from build123d import *

# Parameters (mm, degrees)
SKETCH1_R            = 1.5
BOSS_EXTRUDE1_DEPTH  = 2
SKETCH2_R            = 2
BOSS_EXTRUDE2_DEPTH  = 0.5
SKETCH3_W            = 5
SKETCH3_H            = 5
BOSS_EXTRUDE3_DEPTH  = 10.5
SKETCH4_R            = 1.9
BOSS_EXTRUDE4_DEPTH  = 3.5
BOSS_EXTRUDE5_DEPTH  = 2.5
BOSS_EXTRUDE9_DEPTH  = 2
SKETCH8_R            = 2
BOSS_EXTRUDE10_DEPTH = 5
BOSS_EXTRUDE12_START = -3.5
BOSS_EXTRUDE12_DEPTH = 3.5
CUT_EXTRUDE1_START   = -3.5
CUT_EXTRUDE1_DEPTH   = 3.5
CUT_EXTRUDE4_START   = -2.25
CUT_EXTRUDE4_DEPTH   = 2.25
SKETCH14_R           = 2
SKETCH14_R_2         = 1.5
CUT_EXTRUDE5_DEPTH   = 3.25
BOSS_EXTRUDE13_START = 0.5
SKETCH15_R           = 2
SKETCH15_R_2         = 1.5
BOSS_EXTRUDE13_DEPTH = 0.5
BOSS_EXTRUDE14_START = 0.5
SKETCH17_R           = 1.5
BOSS_EXTRUDE14_DEPTH = 0.5


# Read off the part's stored shape, not the designer's step: Cut-Extrude4
with BuildPart() as part:
    # Sketch1 → Boss-Extrude1 (new body)
    with BuildSketch(Plane(origin=(0, 0, 0), x_dir=(1, 0, 0), z_dir=(0, 1, 0))):
        with Locations(Location((0, 0, 0), (0, 0, 270))):
            Circle(SKETCH1_R)
    extrude(amount=BOSS_EXTRUDE1_DEPTH)

    # Sketch2 → Boss-Extrude2 (add)
    with BuildSketch(Plane(origin=(0, 2, 0), x_dir=(1, 0, 0), z_dir=(0, 1, 0))):
        with Locations(Location((0, 0, 0), (0, 0, 270))):
            Circle(SKETCH2_R)
    extrude(amount=BOSS_EXTRUDE2_DEPTH)

    # Sketch3 → Boss-Extrude3 (add)
    with BuildSketch(Plane(origin=(0, 2.5, 0), x_dir=(1, 0, 0), z_dir=(0, 1, 0))):
        Rectangle(SKETCH3_W, SKETCH3_H)
    extrude(amount=BOSS_EXTRUDE3_DEPTH)

    # Sketch4 → Boss-Extrude4 (add)
    with BuildSketch(Plane(origin=(0, 13, 0), x_dir=(1, 0, 0), z_dir=(0, 1, 0))):
        with Locations(Location((0, 0, 0), (0, 0, 270))):
            Circle(SKETCH4_R)
    extrude(amount=BOSS_EXTRUDE4_DEPTH)

    # Sketch5 → Boss-Extrude5 (add)
    with BuildSketch(Plane(origin=(0, 16.5, 0), x_dir=(1, 0, 0), z_dir=(0, 1, 0))):
        with BuildLine():
            Line((1.549193338, -1.1), (-1.549193338, -1.1))
            ThreePointArc((-1.549193338, -1.1), (0, 1.9), (1.549193338, -1.1))
        make_face()
    extrude(amount=BOSS_EXTRUDE5_DEPTH)

    # Sketch7 → Boss-Extrude9 (add)
    with BuildSketch(Plane(origin=(2.5, 0, 0), x_dir=(0, 0, -1), z_dir=(1, 0, 0))):
        with BuildLine():
            ThreePointArc((-2.5, 3.469223594), (-2.090990258, 2.909009742), (-1.530776406, 2.5))
            Line((-1.530776406, 2.5), (0.530776406, 2.5))
            ThreePointArc((0.530776406, 2.5), (1.090990258, 6.090990258), (-2.5, 5.530776406))
            Line((-2.5, 5.530776406), (-2.5, 3.469223594))
        make_face()
    boss_extrude9 = extrude(amount=BOSS_EXTRUDE9_DEPTH)

    # Sketch8 → Boss-Extrude10 (add)
    with BuildSketch(Plane(origin=(4.5, 0, 0), x_dir=(0, 0, -1), z_dir=(1, 0, 0))):
        with Locations(Location((-0.5, 4.5, 0), (0, 0, 180))):
            Circle(SKETCH8_R)
    boss_extrude10 = extrude(amount=BOSS_EXTRUDE10_DEPTH)

    # Mirror1: Boss-Extrude9, Boss-Extrude10 across plane
    add(boss_extrude9.mirror(Plane(origin=(0, 0, 0), x_dir=(0, 0, 1), z_dir=(1, 0, 0))))
    add(boss_extrude10.mirror(Plane(origin=(0, 0, 0), x_dir=(0, 0, 1), z_dir=(1, 0, 0))))

    # Sketch10 → Boss-Extrude12 (add)
    with BuildSketch(Plane(origin=(0, 16.5, 0), x_dir=(1, 0, 0), z_dir=(0, 1, 0)).offset(BOSS_EXTRUDE12_START)):
        with BuildLine():
            ThreePointArc((-1.549193338, -1.1), (0, -1.9), (1.549193338, -1.1))
            Line((1.549193338, -1.1), (-1.549193338, -1.1))
        make_face()
    extrude(amount=BOSS_EXTRUDE12_DEPTH)

    # Sketch11 → Cut-Extrude1 (cut)
    with BuildSketch(Plane(origin=(0, 16.5, 0), x_dir=(1, 0, 0), z_dir=(0, 1, 0)).offset(CUT_EXTRUDE1_START)):
        with BuildLine():
            Line((-1.549193338, -1.1), (1.549193338, -1.1))
            ThreePointArc((1.549193338, -1.1), (0, -1.9), (-1.549193338, -1.1))
        make_face()
    extrude(amount=CUT_EXTRUDE1_DEPTH, mode=Mode.SUBTRACT)

    # Cut-Extrude4 outline → Cut-Extrude4 (cut)
    with BuildSketch(Plane(origin=(9.5, 0, 0), x_dir=(0, 0, -1), z_dir=(1, 0, 0)).offset(CUT_EXTRUDE4_START)):
        with BuildLine():
            ThreePointArc((0.5, 2.767949192), (1.5, 4.5), (0.5, 6.232050808))
            Line((0.5, 6.232050808), (0.5, 2.767949192))
        make_face()
    extrude(amount=CUT_EXTRUDE4_DEPTH, mode=Mode.SUBTRACT)

    # Sketch14 → Cut-Extrude5 (cut)
    with BuildSketch(Plane.ZY.offset(9.5)):
        with Locations((0.5, 4.5)):
            Circle(SKETCH14_R)
        with Locations((0.5, 4.5)):
            Circle(SKETCH14_R_2, mode=Mode.SUBTRACT)
    extrude(amount=-CUT_EXTRUDE5_DEPTH, mode=Mode.SUBTRACT)

    # Sketch15 → Boss-Extrude13 (add)
    with BuildSketch(Plane.ZY.offset(6.25).offset(BOSS_EXTRUDE13_START)):
        with Locations((0.5, 4.5)):
            Circle(SKETCH15_R)
        with Locations((0.5, 4.5)):
            Circle(SKETCH15_R_2, mode=Mode.SUBTRACT)
    extrude(amount=-BOSS_EXTRUDE13_DEPTH)

    # Sketch17 → Boss-Extrude14 (add)
    with BuildSketch(Plane.ZY.offset(9.5).offset(BOSS_EXTRUDE14_START)):
        with Locations((0.5, 4.5)):
            Circle(SKETCH17_R)
    extrude(amount=-BOSS_EXTRUDE14_DEPTH)


solid = part.part
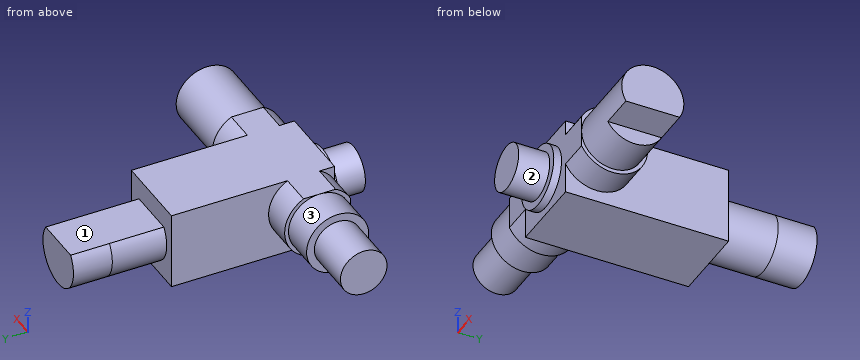
Read the model definition and answer for the solid it produces. Units are mm, in the model's axes. Face numbers are marked on the shaded views. A direction names the side the tool comes from. Round coordinates to 2 decimals unless told otherwise and drop trailing zeros. Order: outer loops, then holes, each group sorted by start corner. A loop starts at its lowest first (then second) coordinate and runs counter-clockwise, first axis right, second up.
1) For the marked faces 1, 2 and 3, determine the directions among +Z, -Z, +X, -X, +Y, -Y from which every point of the face is accessible in a straight line to the end or side of a thin tool.
2) Straight lines are drawn through the part: L1, parallel to X at y = 10, z = 0.65; L2, parallel to Y at x = 5.75, z = 0.5; L3, parallel to X at y = 15.75, z = -0.1. For each, find the intervals that lie inside material, in ascending order.
3) The part is cut by section A-A on x = -1.25. Write down the section's boundary in (y, z).
4) Flat-ended cylindrical pins translate along their axes: pin 1 (1.5 mm diameter, centred on y = 5.5, z = -1, fed in from +X); pin 2 (2.5 mm diameter, centred on x = 9, y = 4.5, fed in from -Z); pin 3 (0.5 mm diameter, centred on y = 3.5, z = -1, fed in from +X); pin 4 (0.8 mm diameter, centred on y = 3, z = 2, fed in from -X). Find the tip coordinate at first contact, or state that the pin passes through.
5) The part is cut by section D-D on x = 4.75. Write down the section's boundary in (y, z).
6) The part is cut by section C-C on y = 8. Write down the section's boundary in (x, z), plus the area to 3 significant figures.
Resolved:
1. face 1: +Z, +X, -X, +Y
1. face 2: -Y
1. face 3: -X
2. L1: x = -2.5 to 2.5
2. L2: y = 2.5 to 6.5
2. L3: x = -1.9 to 1.9
3. outline: (0, -0.83) - (2, -0.83) - (2, -1.56) - (2.5, -1.56) - (2.5, -2.5) - (13, -2.5) - (13, -1.43) - (19, -1.43) - (19, 1.1) - (13, 1.1) - (13, 2.5) - (2.5, 2.5) - (2.5, 1.56) - (2, 1.56) - (2, 0.83) - (0, 0.83) - close
4. pin 1: stops at x = 9.5
4. pin 2: stops at z = -0.5
4. pin 3: stops at x = 7.25
4. pin 4: stops at x = -6.75
5. outline: circle Ø4 at (4.5, 0.5)
6. outline: (-2.5, -2.5) - (2.5, -2.5) - (2.5, 2.5) - (-2.5, 2.5) - close
6. area: 25.0 mm2
